Part model, mm, in its own coordinate system. Face numbers are marked on the shaded views. A direction names the side the tool comes from. Coordinates: 2 decimals unless noted, no trailing zeros. Loops run counter-clockwise (first coordinate to the right, second up) from the corner with the lowest first, then second, coordinate; pieces in that order, holes last. Notation, with made-up numbers: (-15.5, 62) - (8.5, 62) arc R9 cw to (8.5, 76) - close; hole circle Ø4 at (71.5, -4.75). An arc over 180 degrees is marked (long way). Use a Markdown table: item, result. Add a question column.
1. Band-saw the part on B-B, the plane z = -8.75. Give the cut face in (x, y).
2. Drop flat-ended pins along their axis: pin 1 (6 mm diameter, centred on x = 15, y = 0, fed in from -Z); pin 2 (4 mm diameter, centred on x = 35, y = -35, fed in from +Z); pin 3 (5 mm diameter, centred on x = -26, z = -7, fed in from +Y); pin 4 (1.5 mm diameter, centred on x = -7.5, z = -9.5, fed in from +Y). Give the stop position or say it passes through.
3. Band-saw the part on A-A, the plane y = 0. Count the separate pieces of the cut face and the enclosed holes in it, plus the area to 3 significant figures.
4. Band-saw the part on C-C, the plane z = 7.25. Give the cut face in (x, y).
5. Pull direction X, two halves, no side cores. Call the marked faces 3, 4 and 5: pulls with the +X half, pulls with the -X half, needs draft (parallel to the pull), parting line crosses it, or undercut.
6. 3-axis set-ups, long thin cutter, end or side, ignore diameter. For the marked faces 1 and 2: which of +Z, -Z, +X, -X, +Y, -Y reach the whole face in a straight line?
7. Wall check: probe 1 along Y at (x, z) = (-35, -0.7); probe 2 along Z at (x, y) = (-29.5, 20.5). Give the ranges that are in metal, low to high. Write a range as [from, to].
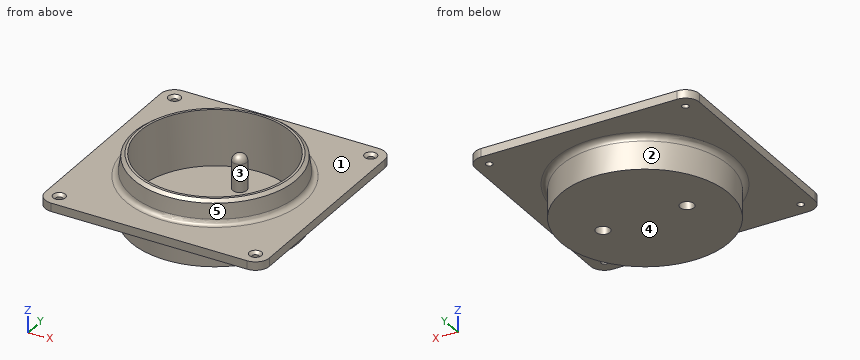
from build123d import *

# Parameters (mm, degrees)
PROFIL_BASE_W                                  = 80
PROFIL_BASE_H                                  = 80
BOSS_EXTRU_1_DEPTH                             = 1.5
CONG_1_R                                       = 5
ESQUISSE2_R                                    = 30
BOSS_EXTRU_2_DEPTH                             = 8
BOSS_EXTRU_2_TAPER                             = 8
BOSS_EXTRU_2_OTHER_WAY_DEPTH                   = 15
ESQUISSE4_R                                    = 26.875673322
ENL_V_MAT_EXTRU_1_DEPTH                        = 20
DIAM_TRE_DU_PER_AGE_0_15_5_1_D                 = 5
ESQUISSE8_R                                    = 2.5
BOSS_EXTRU_3_DEPTH                             = 10
R_VOLUTION1_ANGLE                              = 180
CHANFREIN1_SIZE                                = 1
CHANFREIN1_SIZE_2                              = 1.174957012
CONG_2_R                                       = 2
FRAISAGE_POUR_VIS_T_TE_FRAIS_E_M21_D           = 2.4
FRAISAGE_POUR_VIS_T_TE_FRAIS_E_M21_CSINK_D     = 4.4
FRAISAGE_POUR_VIS_T_TE_FRAIS_E_M21_CSINK_ANGLE = 90


with BuildPart() as part:
    # Profil Base → Boss.-Extru.1 (new, symmetric)
    with BuildSketch(Plane.XY):
        Rectangle(PROFIL_BASE_W, PROFIL_BASE_H)
    extrude(amount=BOSS_EXTRU_1_DEPTH, both=True)

    # Congé1
    cong_1_edges = [part.edges().sort_by_distance(p)[0] for p in [
        (40, -40, 0),
        (-40, -40, 0),
        (-40, 40, 0),
        (40, 40, 0),
    ]]
    fillet(cong_1_edges, radius=CONG_1_R)

    # Esquisse2 → Boss.-Extru.2 (add)
    with BuildSketch(Plane.XY.offset(1.5)):
        Circle(ESQUISSE2_R)
    extrude(amount=BOSS_EXTRU_2_DEPTH, taper=BOSS_EXTRU_2_TAPER)

    # Esquisse2 → Boss.-Extru.2 other way (add)
    with BuildSketch(Plane.XY.offset(1.5)):
        Circle(ESQUISSE2_R)
    extrude(amount=-BOSS_EXTRU_2_OTHER_WAY_DEPTH)

    # Esquisse4 → Enlèv. mat.-Extru.1 (cut)
    with BuildSketch(Plane.XY.offset(9.5)):
        Circle(ESQUISSE4_R)
    extrude(amount=-ENL_V_MAT_EXTRU_1_DEPTH, mode=Mode.SUBTRACT)

    # Diamètre du perçage Ø0.15 (5)1 (through all)
    with Locations(Plane.XY.offset(-10.5)):
        with Locations((-15, 0), (15, 0)):
            Hole(DIAM_TRE_DU_PER_AGE_0_15_5_1_D / 2)

    # Esquisse8 → Boss.-Extru.3 (add)
    with BuildSketch(Plane.XY.offset(-10.5)):
        with Locations((0, 15)):
            Circle(ESQUISSE8_R)
    extrude(amount=BOSS_EXTRU_3_DEPTH)

    # Esquisse9 → Révolution1 (revolve)
    with BuildSketch(Plane.XY.offset(-0.5)):
        with BuildLine():
            Line((0, 17.5), (0, 12.5))
            ThreePointArc((0, 12.5), (2.5, 15), (0, 17.5))
        make_face()
    revolve(axis=Axis((0, 17.5, -0.5), (0, -1, 0)), revolution_arc=R_VOLUTION1_ANGLE)

    # Chanfrein1
    # the kernel refuses this chamfer: 1.174957012, 1 mm, written as the material it takes off along each edge
    with BuildSketch(Plane(origin=(0, 0, 9.5), x_dir=(1, 0, 0), z_dir=(0, 1, 0))) as chanfrein1_piece_1:
        Polygon((28.875673322 + CHANFREIN1_SIZE * 0.13917310096, CHANFREIN1_SIZE * 0.990268068742), (28.875673322 - CHANFREIN1_SIZE_2, 0), (28.875673322, 0), align=None)
    revolve(axis=Axis((0, 0, 9.5), (0, 0, -1)), mode=Mode.SUBTRACT)

    # Congé2
    cong_2_edges = [part.edges().sort_by_distance(p)[0] for p in [
        (-30, 0, -1.5),
        (-30, 0, 1.5),
    ]]
    fillet(cong_2_edges, radius=CONG_2_R)

    # Fraisage pour vis à tête fraisée M21 (through all)
    with Locations(Plane.XY.offset(1.5)):
        with Locations((-35, 35), (35, 35), (-35, -35), (35, -35)):
            CounterSinkHole(FRAISAGE_POUR_VIS_T_TE_FRAIS_E_M21_D / 2, FRAISAGE_POUR_VIS_T_TE_FRAIS_E_M21_CSINK_D / 2, counter_sink_angle=FRAISAGE_POUR_VIS_T_TE_FRAIS_E_M21_CSINK_ANGLE)


solid = part.part
Geometry check:
| question | item | result |
|---|---|---|
| 1 | outline | circle Ø60 at (0, 0); circle Ø5 at (0, 15); hole circle Ø53.75 at (0, 0) |
| 2 | pin 1 | stops at z = -13.5 |
| 2 | pin 2 | stops at z = 1.3 |
| 2 | pin 3 | stops at y = 18.65 |
| 2 | pin 4 | stops at y = 29.23 |
| 3 | separate pieces | 3 |
| 3 | enclosed holes | 0 |
| 3 | area | 328 mm^2 |
| 4 | outline | circle Ø58.38 at (0, 0); hole circle Ø53.75 at (0, 0) |
| 5 | face 3 | undercut |
| 5 | face 4 | needs draft |
| 5 | face 5 | parting line crosses it |
| 6 | face 1 | +Z |
| 6 | face 2 | -Z |
| 7 | probe 1 | y = [-40, -36.2], [-33.8, 33.8], [36.2, 40] |
| 7 | probe 2 | z = [-1.5, 1.5] |
